Part model, mm, in its own coordinate system. Face numbers are marked on the shaded views. A direction names the side the tool comes from. Give positions to 0.01 mm unless a question says otherwise; leave off trailing zeros. Write each loop counter-clockwise with the first axis right and the second up, starting at its lowest first coordinate (ties: lowest second). Pieces come first, ordered by that corner, then holes. Notation, with made-up numbers: M -31,-29.75 L -15,-29.75 A9 cw -15,-16.75 Z; hole C -37.5,2.25 d5. An arc over 180 degrees is marked long. Use a Markdown table: item, result.
```python
from build123d import *

# Parameters (mm, degrees)
DODANIE_WYCI_GNI_CIE1_DEPTH = 5
SZKIC3_R                    = 24
DODANIE_WYCI_GNI_CIE2_DEPTH = 25
OTW_R_36_0_36_1_D           = 36


with BuildPart() as part:
    # Szkic2 → Dodanie-wyciągnięcie1 (new body)
    with BuildSketch(Plane(origin=(0, 0, 0), x_dir=(0, 0, -1), z_dir=(1, 0, 0))):
        with BuildLine():
            ThreePointArc((0, 57), (0.878679656, 59.121320344), (3, 60))
            Line((3, 60), (57, 60))
            ThreePointArc((57, 60), (59.121320344, 59.121320344), (60, 57))
            Line((60, 57), (60, 3))
            ThreePointArc((60, 3), (59.121320344, 0.878679656), (57, 0))
            Line((57, 0), (3, 0))
            ThreePointArc((3, 0), (0.878679656, 0.878679656), (0, 3))
            Line((0, 3), (0, 57))
        make_face()
    extrude(amount=DODANIE_WYCI_GNI_CIE1_DEPTH)

    # Szkic3 → Dodanie-wyciągnięcie2 (add)
    with BuildSketch(Plane(origin=(5, 0, 0), x_dir=(0, 0, -1), z_dir=(1, 0, 0))):
        with Locations((30, 30)):
            Circle(SZKIC3_R)
    extrude(amount=DODANIE_WYCI_GNI_CIE2_DEPTH)

    # Otwór Ø36.0 (36)1 (through all)
    with Locations(Plane(origin=(30, 0, 0), x_dir=(0, 0, -1), z_dir=(1, 0, 0))):
        with Locations((30, 30)):
            Hole(OTW_R_36_0_36_1_D / 2)


solid = part.part
```
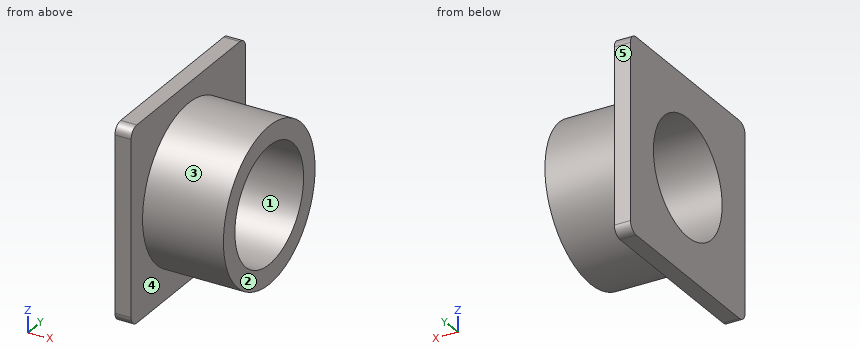
1. Cut at C-C, the plane x = 12.5. Give the cut face in (y, z).
Findings below:
| item | result |
|---|---|
| outline | C 30,-30 d48; hole C 30,-30 d36 |
2. Drop flat-ended pins along their axis: P1, Ø1.5, axis at x = 22, y = 35.5, coming from the +Z side; P2, Ø1.5, axis at x = 17, y = 22, coming from the +Z side; P3, Ø10, axis at x = 10.5, z = -52, coming from the +Y side. Give the stop position or say it passes through.
Findings below:
| item | result |
|---|---|
| P1 | z = -6.47 |
| P2 | z = -7.12 |
| P3 | y = 46.94 |
3. Two-plate mould, pull along Z, no slides. Class the marked faces 1, 2 and 3: released by +Z, released by -Z, zero draft, split by the parting line, or undercut.
Findings below:
| item | result |
|---|---|
| face 1 | undercut |
| face 2 | zero draft |
| face 3 | split by the parting line |
4. Cut at A-A, the plane y = 30. Give the cut face in (x, z), then the cut area to 3 significant figures.
Findings below:
| item | result |
|---|---|
| outline | M 0,-60 L 5,-60 L 5,-54 L 30,-54 L 30,-48 L 0,-48 Z; M 0,-12 L 30,-12 L 30,-6 L 5,-6 L 5,0 L 0,0 Z |
| area | 420 mm2 |
5. Cut at B-B, the plane z = -30. Give the cut face in (x, y), then the cut area to 3 significant figures.
Findings below:
| item | result |
|---|---|
| outline | M 0,0 L 5,0 L 5,6 L 30,6 L 30,12 L 0,12 Z; M 0,48 L 30,48 L 30,54 L 5,54 L 5,60 L 0,60 Z |
| area | 420 mm2 |
6. Cut at D-D, the plane z = -4.5. Give the cut face in (x, y), then the cut area to 3 significant figures.
Findings below:
| item | result |
|---|---|
| outline | M 0,0 L 5,0 L 5,60 L 0,60 Z |
| area | 300 mm2 |
7. Drill centre lines: L1, parallel to Y at x = 15.75, z = -30; L2, parallel to X at y = 43, z = -2.5; L3, parallel to Y at x = 20.25, z = -27.5. Where is each one in solid material? Low to high.
Findings below:
| item | result |
|---|---|
| L1 | 6 to 12, 48 to 54 |
| L2 | 0 to 5 |
| L3 | 6.13 to 12.17, 47.83 to 53.87 |
8. Tool access for the marked faces 4 and 5: list every direction of +Z, -Z, +X, -X, +Y, -Y with a clear straight run to the whole face (end or side of a thin tool).
Findings below:
| item | result |
|---|---|
| face 4 | +X |
| face 5 | +Z, -Z, +X, -X, +Y |
